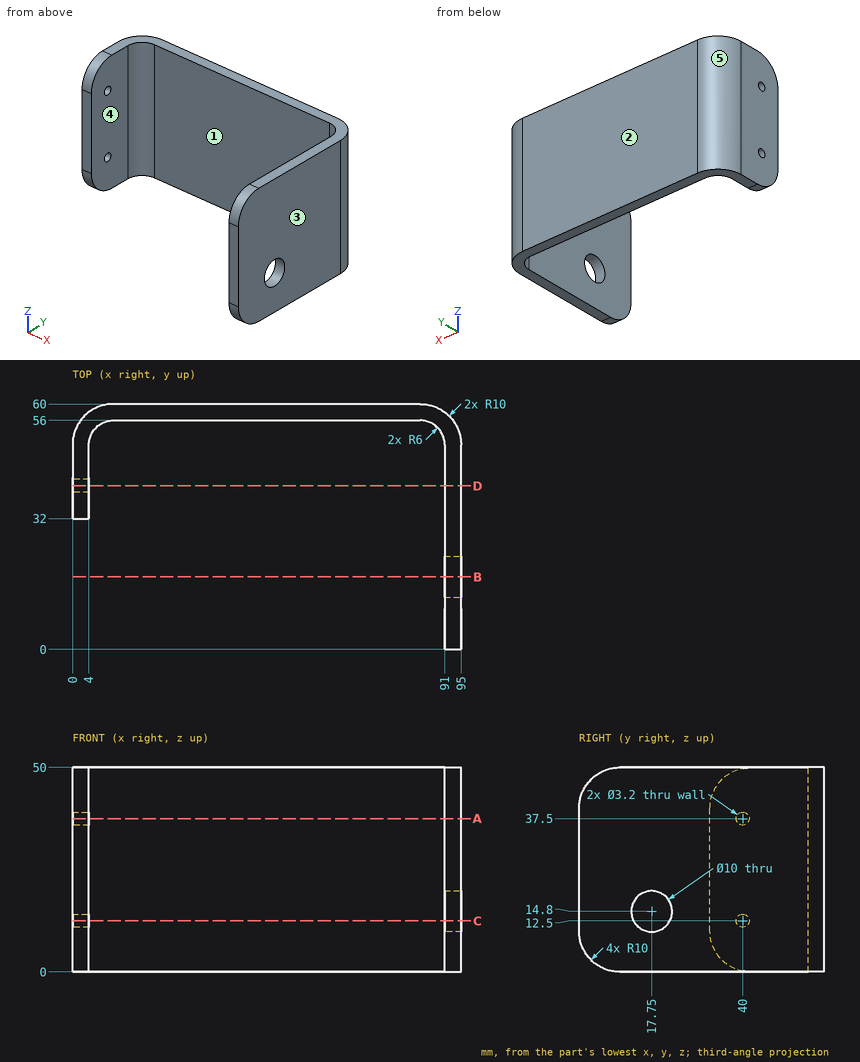
Study the drawing (mm; zero at the part's minimum x, y, z) and answer. A direction names the side the tool comes from. Coordinates: 2 decimals unless noted, no trailing zeros. Write each loop counter-clockwise with the first axis right and the second up, starting at its lowest first coordinate (ties: lowest second). Pieces come first, ordered by that corner, then holes.
Q1. Section C-C, the plane z = 12.5 is taken. Write down the section's boundary in (x, y), then the cut area to 3 significant figures.
Returned:
outline: (0, 32) - (4, 32) - (4, 38.4) - (0, 38.4) - close; (0, 41.6) - (4, 41.6) - (4, 50) arc R6 cw to (10, 56) - (85, 56) arc R6 cw to (91, 50) - (91, 22.19) - (95, 22.19) - (95, 50) arc R10 ccw to (85, 60) - (10, 60) arc R10 ccw to (0, 50) - close; (91, 0) - (95, 0) - (95, 13.31) - (91, 13.31) - close
area: 624 mm2
Q2. Section D-D, the plane y = 40 is taken. Write down the section's boundary in (x, z), then the cut area to 3 significant figures.
Returned:
outline: (0, 0.2) - (4, 0.2) - (4, 10.9) - (0, 10.9) - close; (0, 14.1) - (4, 14.1) - (4, 35.9) - (0, 35.9) - close; (0, 39.1) - (4, 39.1) - (4, 49.8) - (0, 49.8) - close; (91, 0) - (95, 0) - (95, 50) - (91, 50) - close
area: 373 mm2
Q3. Section A-A, the plane z = 37.5 is taken. Write down the section's boundary in (x, y), then the cut area to 3 significant figures.
Returned:
outline: (0, 32) - (4, 32) - (4, 38.4) - (0, 38.4) - close; (0, 41.6) - (4, 41.6) - (4, 50) arc R6 cw to (10, 56) - (85, 56) arc R6 cw to (91, 50) - (91, 0) - (95, 0) - (95, 50) arc R10 ccw to (85, 60) - (10, 60) arc R10 ccw to (0, 50) - close
area: 660 mm2
Q4. Given P1, Ø1.5, axis at x = 27.5, z = 25.5, coming from the -Y side; P2, Ø1.2, axis at x = 2.5, z = 19.5, coming from the -Y side; P3, Ø3, axis at y = 40, z = 37.5, coming from the -X side, each flat-ended and moving along its own axis, determine where each tip first touches the part or whether it passes through.
Returned:
P1: stops at y = 56
P2: stops at y = 32
P3: stops at x = 91
Q5. The mould has two halves that part along X. Classify the marked faces 1, 2 and 3: released by +X, released by -X, zero draft, split by the parting line, or undercut.
Returned:
face 1: undercut
face 2: zero draft
face 3: released by +X
Q6. Find the intervals of material crossed by line 1 along X through (y, z) = (35.5, 11); line 2 along Y through (x, z) = (68.5, 7); line 3 along X through (y, z) = (7.5, 32.5), in increasing order.
Returned:
line 1: x = 0 to 4, 91 to 95
line 2: y = 56 to 60
line 3: x = 91 to 95
Q7. Which of the six approach directions +Z, -Z, +X, -X, +Y, -Y give full straight-line access (tool end or side, diameter ignored) to the marked faces 4 and 5?
Returned:
face 4: +Z, -Z, -Y
face 5: +Z, -Z, -X, +Y
Q8. Section B-B, the plane y = 17.75 is taken. Write down the section's boundary in (x, z).
Returned:
outline: (91, 0) - (95, 0) - (95, 9.8) - (91, 9.8) - close; (91, 19.8) - (95, 19.8) - (95, 50) - (91, 50) - close
